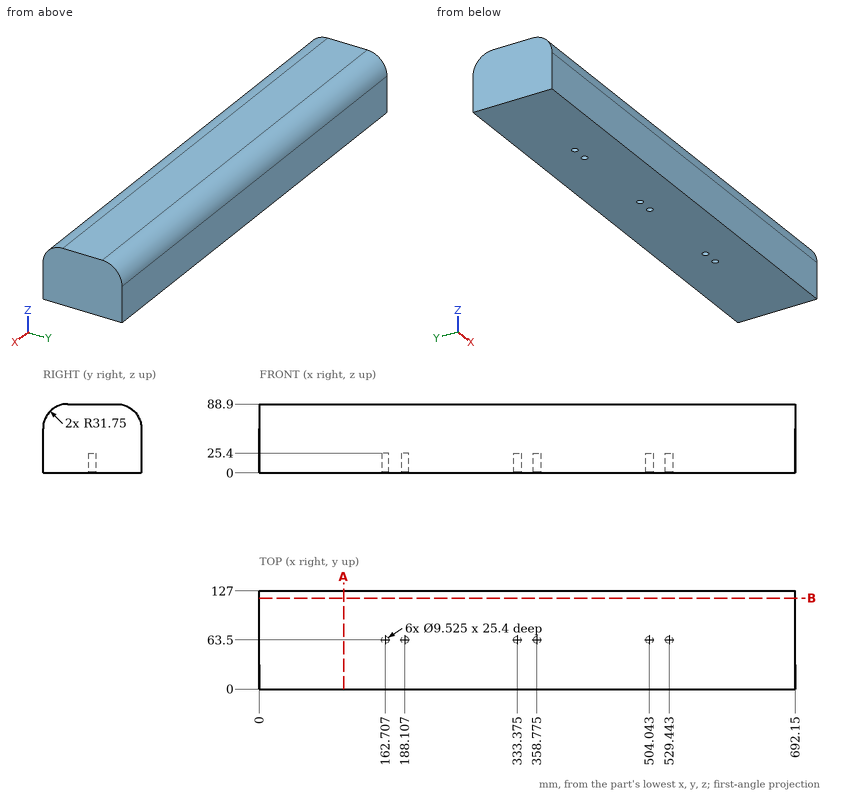
Verification items for this drawing (mm, ordinates from the low corner). Round coordinates to 2 decimals unless told otherwise and drop trailing zeros. Order: outer loops, then holes, each group sorted by start corner. A loop starts at its lowest first (then second) coordinate and runs counter-clockwise, first axis right, second up.
1) Cross-section at A-A, the plane x = 109. Record the cut outline in (y, z), plus the area to 3 significant figures.
Geometry says:
outline: (0, 0) - (127, 0) - (127, 57.15) arc R31.75 ccw to (95.25, 88.9) - (31.75, 88.9) arc R31.75 ccw to (0, 57.15) - close
area: 10,900 mm2
2) Cross-section at B-B, the plane y = 117.5. Record the cut outline in (x, z), plus the area to 3 significant figures.
Geometry says:
outline: (0, 0) - (692.15, 0) - (692.15, 79.8) - (0, 79.8) - close
area: 55,200 mm2
3) Material ranges on line 1 (Y direction, x = 360, z = 15.5); line 2 (Y direction, x = 653, z = 60); line 3 (Y direction, x = 614.5, z = 60.5), recorded low to high.
Geometry says:
line 1: y = 0 to 58.9, 68.1 to 127
line 2: y = 0.13 to 126.87
line 3: y = 0.18 to 126.82
4) Depth check by flat-ended pin: pin 1 (8 mm diameter, centred on x = 238.5, y = 40, fed in from -Z); pin 2 (3 mm diameter, centred on x = 530.5, y = 64, fed in from -Z); pin 3 (4 mm diameter, centred on x = 334.5, z = 71.5, fed in from -Y); pin 4 (1.5 mm diameter, centred on x = 408.5, y = 29.5, fed in from +Z). Enter the tip coordinate at first touch or a pass-through.
Geometry says:
pin 1: stops at z = 0
pin 2: stops at z = 25.4
pin 3: stops at y = 2.5
pin 4: stops at z = 88.86
